```python
from build123d import *

# Parameters (mm, degrees)
SKETCH_1_W      = 39
SKETCH_1_H      = 10
SKETCH_1_R      = 1.6
SKETCH_1_W_2    = 2
SKETCH_1_H_2    = 5
EXTRUDE_1_DEPTH = 3
SKETCH_2_W      = 39
SKETCH_2_H      = 15
SKETCH_2_R      = 1.6
EXTRUDE_2_DEPTH = 3
CHAMFER_1_SIZE  = 1.5
FILLET_1_R      = 2


with BuildPart() as part:
    # ｽｹｯﾁ1 → ﾎﾞｽ - 押し出し1 (new body)
    with BuildSketch(Plane.XY):
        with Locations((9.5, 0)):
            Rectangle(SKETCH_1_W, SKETCH_1_H)
        Circle(SKETCH_1_R, mode=Mode.SUBTRACT)
        with Locations((19, 0)):
            Circle(SKETCH_1_R, mode=Mode.SUBTRACT)
        with Locations((5, 0)):
            Rectangle(SKETCH_1_W_2, SKETCH_1_H_2, mode=Mode.SUBTRACT)
        with Locations((14, 0)):
            Rectangle(SKETCH_1_W_2, SKETCH_1_H_2, mode=Mode.SUBTRACT)
    extrude(amount=EXTRUDE_1_DEPTH)

    # ｽｹｯﾁ2 → ﾎﾞｽ - 押し出し2 (add)
    with BuildSketch(Plane.XZ.offset(5)):
        with Locations((9.5, 7.5)):
            Rectangle(SKETCH_2_W, SKETCH_2_H)
        with Locations((-5.5, 7.5)):
            Circle(SKETCH_2_R, mode=Mode.SUBTRACT)
        with Locations((24.5, 7.5)):
            Circle(SKETCH_2_R, mode=Mode.SUBTRACT)
    extrude(amount=EXTRUDE_2_DEPTH)

    # 面取り1
    chamfer_1_edges = [part.edges().sort_by_distance(p)[0] for p in [
        (9.5, -5, 3),
    ]]
    chamfer(chamfer_1_edges, length=CHAMFER_1_SIZE)

    # ﾌｨﾚｯﾄ1
    fillet_1_edges = [part.edges().sort_by_distance(p)[0] for p in [
        (29, -6.5, 15),
        (-10, -6.5, 15),
        (29, 5, 1.5),
        (-10, 5, 1.5),
    ]]
    fillet(fillet_1_edges, radius=FILLET_1_R)


solid = part.part
```
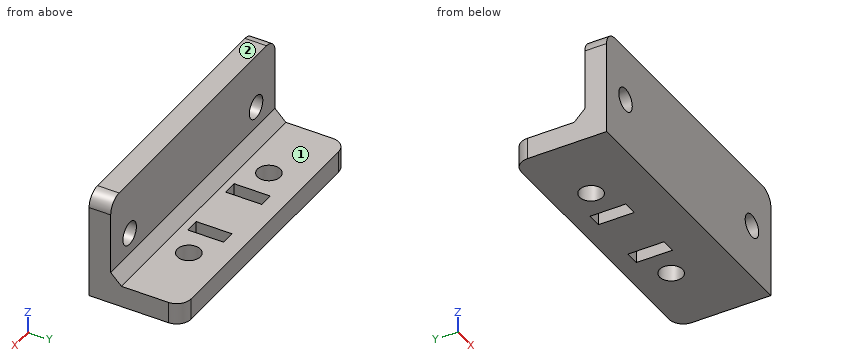
Design review of the part built by this model. Coordinates are the model's own, in mm. Face numbers are marked on the shaded views. A direction names the side the tool comes from. Give positions to 0.01 mm unless a question says otherwise; leave off trailing zeros. Write each loop counter-clockwise with the first axis right and the second up, starting at its lowest first coordinate (ties: lowest second). Pieces come first, ordered by that corner, then holes. Notation, with made-up numbers: (19, -6.5) - (27, -6.5) arc R22 ccw to (27, 19.5) - close; hole circle Ø2 at (80, 41). An arc over 180 degrees is marked (long way). Return JSON: item names as keys, results as strings. Group by question number.
(1) We need section B-B, the plane x = 0. Give the boundary of the cut face in (y, z).
(2) Insertion check: pin 1 (6 mm diameter, centred on y = -0.5, z = 7, fed in from -X); pin 2 (2.5 mm diameter, centred on x = 0.5, y = -1, fed in from +Z); pin 3 (5 mm diameter, centred on x = 7.5, y = -1.5, fed in from +Z); pin 4 (3.5 mm diameter, centred on x = 24.5, z = 7.5, fed in from +Y). Each pin has a flat end and moves straight along its axis. Give the tip position at first contact, or say it passes through.
(3) To check wall thickness, follow probe 1 along Y at (x, z) = (0, 2); probe 2 along X at (y, z) = (-6, 7.75); probe 3 along Z at (x, y) = (-5.5, -5.7). State the ranges of each line that lie inside material, in increasing order.
(4) We need section D-D, the plane y = -0.75. Give the boundary of the cut face in (x, z), then the cut area to 3 significant figures.
(5) We need section C-C, the plane z = 2.25. Give the boundary of the cut face in (x, y).
(6) Machinability: for the marked faces 1 and 2, which of the approach directions +Z, -Z, +X, -X, +Y, -Y give a long, thin tool a straight path to every point of the face, cutting with its end or side? Answer none if there is none.
(7) We need section A-A, the plane z = 7.5. Give the boundary of the cut face in (x, y), then the cut area to 3 significant figures.
Reported:
{
 "1": {"outline": "(-8, 0) - (-1.6, 0) - (-1.6, 3) - (-3.5, 3) - (-5, 4.5) - (-5, 15) - (-8, 15) - close; (1.6, 0) - (5, 0) - (5, 3) - (1.6, 3) - close"},
 "2": {"pin 1": "passes through", "pin 2": "stops at z = 3", "pin 3": "stops at z = 3.5", "pin 4": "stops at y = -5"},
 "3": {"probe 1": "y = -8 to -1.6, 1.6 to 5", "probe 2": "x = -10 to -7.08, -3.92 to 22.92, 26.08 to 29", "probe 3": "z = 0 to 5.9, 9.1 to 15"},
 "4": {"outline": "(-10, 0) - (-1.41, 0) - (-1.41, 3) - (-10, 3) - close; (1.41, 0) - (4, 0) - (4, 3) - (1.41, 3) - close; (6, 0) - (13, 0) - (13, 3) - (6, 3) - close; (15, 0) - (17.59, 0) - (17.59, 3) - (15, 3) - close; (20.41, 0) - (29, 0) - (29, 3) - (20.41, 3) - close", "area": "88.0 mm2"},
 "5": {"outline": "(-10, -8) - (29, -8) - (29, 3) arc R2 ccw to (27, 5) - (-8, 5) arc R2 ccw to (-10, 3) - close; hole circle Ø3.2 at (0, 0); hole (4, -2.5) - (6, -2.5) - (6, 2.5) - (4, 2.5) - close; hole (13, -2.5) - (15, -2.5) - (15, 2.5) - (13, 2.5) - close; hole circle Ø3.2 at (19, 0)"},
 "6": {"face 1": "+Z, +X, -X, +Y", "face 2": "+Z, +X, -X, +Y, -Y"},
 "7": {"outline": "(-10, -8) - (-7.1, -8) - (-7.1, -5) - (-10, -5) - close; (-3.9, -8) - (22.9, -8) - (22.9, -5) - (-3.9, -5) - close; (26.1, -8) - (29, -8) - (29, -5) - (26.1, -5) - close", "area": "97.8 mm2"}
}
